The model under review builds one solid part; all positions refer to its coordinate system, in mm. Give positions to 0.01 mm unless a question says otherwise; leave off trailing zeros. Order: outer loops, then holes, each group sorted by start corner. A loop starts at its lowest first (then second) coordinate and runs counter-clockwise, first axis right, second up. Notation, with made-up numbers: (72, 60) - (113, 60) arc R38 ccw to (113, 99) - close; hole circle Ø5 at (-10.75, 10). An arc over 180 degrees is marked (long way). Use CSV: the item, a comma, the result in double quotes. Start each with the question number.
```python
from build123d import *

# Parameters (mm, degrees)
SKETCH_1_W          = 50
SKETCH_1_H          = 50
EXTRUDE_1_DEPTH     = 2
SKETCH_2_R          = 1.6
CUT_EXTRUDE_1_DEPTH = 10
SKETCH_3_W          = 76.549088161
SKETCH_3_H          = 63.496312915
CUT_EXTRUDE_3_DEPTH = 10


with BuildPart() as part:
    # ｽｹｯﾁ1 → ﾎﾞｽ - 押し出し1 (new body)
    with BuildSketch(Plane.XY):
        Rectangle(SKETCH_1_W, SKETCH_1_H)
    extrude(amount=EXTRUDE_1_DEPTH)

    # ｽｹｯﾁ2 → ｶｯﾄ - 押し出し1 (cut)
    with BuildSketch(Plane.XY.offset(2)):
        Circle(SKETCH_2_R)
        with Locations((0, -9.51)):
            Circle(SKETCH_2_R)
        with Locations((0, -19.51)):
            Circle(SKETCH_2_R)
        with Locations((10, 0)):
            Circle(SKETCH_2_R)
    extrude(amount=-CUT_EXTRUDE_1_DEPTH, mode=Mode.SUBTRACT)

    # ｽｹｯﾁ3 → ｶｯﾄ - 押し出し3 (cut)
    with BuildSketch(Plane.XY.offset(2)):
        with Locations((-0.951764861, 3.501134841)):
            Rectangle(SKETCH_3_W, SKETCH_3_H)
        Polygon((14.5, -4.5), (4.5, -25), (-4.5, -25), (-4.5, 4.5), (14.5, 4.5), align=None, mode=Mode.SUBTRACT)
    extrude(amount=-CUT_EXTRUDE_3_DEPTH, mode=Mode.SUBTRACT)


solid = part.part
```
1. Mouldability with a two-part tool opening along X and no side actions: class faces 1 (the face through (-4.5, -10, 1)), 2 (the face through (8.4, 0.07, 1.01)), 3 (the face through (14.5, 0, 1)) as pulls with the +X half, pulls with the -X half, needs draft (parallel to the pull), parting line crosses it, or undercut.
2. To check wall thickness, follow L1, parallel to Y at x = 0, z = 0.4; L2, parallel to X at y = 0.25, z = 1; L3, parallel to X at y = 0.5, z = 0.7. State the ranges of each line that lie inside material, in increasing order. Write a range as [from, to].
3. Consider section C-C (x = 10). Give the boundary of the cut face in (y, z) (3 decimals), and give its area (4 significant figures).
4. Consider section D-D (y = 0). Give the boundary of the cut face in (x, z).
5. Consider section A-A (x = 0). Give the boundary of the cut face in (y, z).
6. Consider section B-B (y = -19.51). Give the boundary of the cut face in (x, z).
7. Clearance check with a flat-ended pin moving along its axis: pin 1 (5 mm diameter, centred on x = 0, y = -9.51, fed in from +Z). State where the tip first meets the part, or that it passes through.
Answers follow:
1,face 1,"pulls with the -X half"
1,face 2,"undercut"
1,face 3,"pulls with the +X half"
2,L1,"y = [-25, -21.11], [-17.91, -11.11], [-7.91, -1.6], [1.6, 4.5]"
2,L2,"x = [-4.5, -1.58], [1.58, 8.42], [11.58, 14.5]"
2,L3,"x = [-4.5, -1.52], [1.52, 8.48], [11.52, 14.5]"
3,outline,"(-13.725, 0) - (-1.6, 0) - (-1.6, 2) - (-13.725, 2) - close; (1.6, 0) - (4.5, 0) - (4.5, 2) - (1.6, 2) - close"
3,area,"30.05 mm^2"
4,outline,"(-4.5, 0) - (-1.6, 0) - (-1.6, 2) - (-4.5, 2) - close; (1.6, 0) - (8.4, 0) - (8.4, 2) - (1.6, 2) - close; (11.6, 0) - (14.5, 0) - (14.5, 2) - (11.6, 2) - close"
5,outline,"(-25, 0) - (-21.11, 0) - (-21.11, 2) - (-25, 2) - close; (-17.91, 0) - (-11.11, 0) - (-11.11, 2) - (-17.91, 2) - close; (-7.91, 0) - (-1.6, 0) - (-1.6, 2) - (-7.91, 2) - close; (1.6, 0) - (4.5, 0) - (4.5, 2) - (1.6, 2) - close"
6,outline,"(-4.5, 0) - (-1.6, 0) - (-1.6, 2) - (-4.5, 2) - close; (1.6, 0) - (7.18, 0) - (7.18, 2) - (1.6, 2) - close"
7,pin 1,"stops at z = 2"
